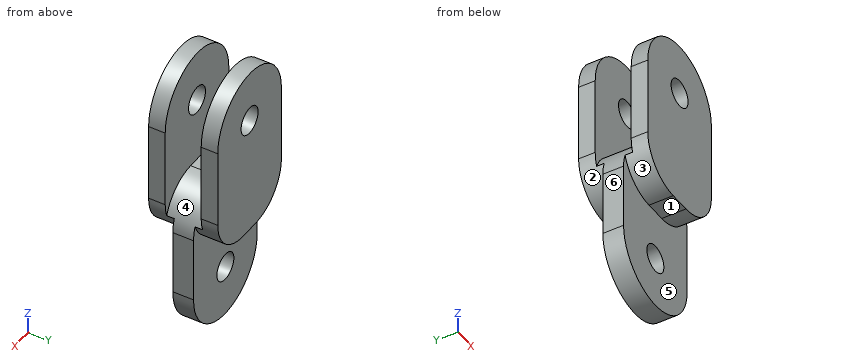
Autodesk Inventor part; units mm, degrees
ref_plane "YZ Plane" through (0, 0, 0) normal (1, 0, 0) x (0, 1, 0)
ref_plane "XZ Plane" through (0, 0, 0) normal (0, 1, 0) x (-1, 0, 0)
ref_plane "XY Plane" through (0, 0, 0) normal (0, 0, 1) x (1, 0, 0)
sketch "Sketch1" plane through (0, 0, 0) normal (0, 1, 0) x (-1, 0, 0)
  line L0 (7.5, 20) -> (-7.5, 20)
  line L1 (-7.5, 20) -> (-7.5, -20)
  line L2 (-7.5, -20) -> (7.5, -20)
  line L3 (7.5, -20) -> (7.5, 20)
  circle A0 centre (0, -12.5) radius 7.5
  circle A1 centre (0, 12.5) radius 7.5
  circle A2 centre (0, 12.5) radius 2
  circle A3 centre (0, -12.5) radius 2
  point P0 (0, 0)
  point P1 (7.5, 0)
  point P2 (0, -20)
  point P3 (7.5, 12.5)
  point P4 (-7.5, 12.5)
  point P5 (-7.5, -12.5)
  point P6 (7.5, -12.5)
  dimension "d0" = 15
  dimension "d2" = 25
  dimension "d3" = 4
  dimension "d4" = 4
extrude "Extrusion1" add sketch "Sketch1" along normal blind 10 contours A1 | L3 A0 L1 A1 | A0
sketch "Sketch2" plane through (7.5, 0, 12.5) normal (1, 0, 0) x (0, 0, -1)
  line L0 (-7.5, 0) -> (-7.5, 10)
  line L1 (-7.5, 7.6) -> (9.5, 7.6)
  line L2 (9.5, 7.6) -> (9.5, 2.4)
  line L3 (9.5, 2.4) -> (-7.5, 2.4)
  line L4 (-7.5, 2.4) -> (-7.5, 7.6)
  point P0 (12.5, 0)
  point P1 (-7.5, 5)
  point P2 (-7.5, 5)
  dimension "d7" = 17
  dimension "d8" = 5.2
extrude "Extrusion2" cut sketch "Sketch2" against normal through all
fillet "Fillet1" radius 6 2 edges at (7.5, 5, 3) (-7.5, 5, 3)
sketch "Sketch4" plane through (7.5, 0, 12.5) normal (1, 0, 0) x (0, 0, -1)
  line L0 (32.5, 0) -> (32.5, 10)
  line L1 (32.5, 6.5) -> (17.5, 6.5)
  line L2 (17.5, 6.5) -> (17.5, 3.5)
  line L3 (17.5, 3.5) -> (32.5, 3.5)
  line L4 (32.5, 3.5) -> (32.5, 6.5)
  line L5 (15.5, 2.4) -> (15.5, 7.6)
  line L6 (0, 0) -> (25, 0)
  line L7 (32.5, 3.5) -> (17.5, 3.5)
  line L8 (17.5, 3.5) -> (17.5, 0)
  line L9 (17.5, 0) -> (32.5, 0)
  line L10 (32.5, 0) -> (32.5, 3.5)
  line L11 (25, 10) -> (0, 10)
  line L12 (32.5, 6.5) -> (17.5, 6.5)
  line L13 (17.5, 6.5) -> (17.5, 10)
  line L14 (17.5, 10) -> (32.5, 10)
  line L15 (32.5, 10) -> (32.5, 6.5)
  point P0 (12.5, 0)
  point P1 (17.5, 5)
  point P2 (15.5, 5)
  point P3 (17.5, 1.75)
  dimension "d15" = 3
  dimension "d16" = 15
extrude "Extrusion4" cut sketch "Sketch4" against normal through all contours L9 L6 L8 L3 L0 | L1 L13 L11 L14 L0
fillet "Fillet2" radius 6 4 edges at (7.5, 1.75, -5) (7.5, 8.25, -5) (-7.5, 1.75, -5) (-7.5, 8.25, -5)
properties part number "coupler"
CAD build for the part. Positions are in the model's coordinates, mm. Face numbers are marked on the shaded views. A direction names the side the tool comes from. Round coordinates to 2 decimals unless told otherwise and drop trailing zeros. Loops run counter-clockwise (first coordinate to the right, second up) from the corner with the lowest first, then second, coordinate; pieces in that order, holes last.
(1) Wall check: line 1 along Z through (x, y) = (0, 0.9); line 2 along Y through (x, z) = (-3, 12.5); line 3 along X through (y, z) = (5.8, -12.5). Give the ranges that are in metal, low to high.
(2) Which spindle directions (+Z, -Z, +X, -X, +Y, -Y) get a long thin tool onto all of the face, cutting with end or side? Do the marked faces 1, 2 and 3. Say none if no direction does.
(3) Cut at A-A (x = 0). Give the cut face in (y, z).
(4) Two-plate mould, pull along Y, no slides. Class the marked faces 4, 5 and 6: +Y half, -Y half, draft (parallel to the pull), parting line (faces both ways), or undercut.
(5) Cut at D-D (x = -3.25). Give the cut face in (y, z), plus the area to 3 significant figures.
(6) Drop flat-ended pins along their axis: pin 1 (6 mm diameter, centred on x = 2.5, z = -13, fed in from -Y); pin 2 (1 mm diameter, centred on x = -5, z = -13, fed in from +Y); pin 3 (0.9 mm diameter, centred on x = 0.5, y = 2, fed in from -Z). Give the stop position or say it passes through.
(7) Cut at B-B (y = 8.75). Give the cut face in (x, z), plus the area to 3 significant figures.
(8) Cut at C-C (z = 4). Give the cut face in (x, y), plus the area to 3 significant figures.
Findings below:
1. line 1: z = -5 to 10.5, 14.5 to 20
1. line 2: y = 0 to 2.4, 7.6 to 10
1. line 3: x = -7.5 to -2, 2 to 7.5
2. face 1: -Z, +X, -X, -Y
2. face 2: -Z, -X, +Y
2. face 3: -Z, -X, -Y
3. outline: (0, -5) - (3.5, -5) - (3.5, -10.5) - (6.5, -10.5) - (6.5, -5) - (10, -5) - (10, 10.5) - (7.6, 10.5) - (7.6, 3) - (2.4, 3) - (2.4, 10.5) - (0, 10.5) - close; (0, 14.5) - (2.4, 14.5) - (2.4, 20) - (0, 20) - close; (3.5, -20) - (6.5, -20) - (6.5, -14.5) - (3.5, -14.5) - close; (7.6, 14.5) - (10, 14.5) - (10, 20) - (7.6, 20) - close
4. face 4: undercut
4. face 5: -Y half
4. face 6: draft
5. outline: (0, -4.74) - (3.5, -4.74) - (3.5, -19.26) - (6.5, -19.26) - (6.5, -4.74) - (10, -4.74) - (10, 19.26) - (7.6, 19.26) - (7.6, 2.74) - (2.4, 2.74) - (2.4, 19.26) - (0, 19.26) - close
5. area: 198 mm2
6. pin 1: stops at y = 3.5
6. pin 2: stops at y = 6.5
6. pin 3: stops at z = -5
7. outline: (-7.5, 1) arc R6 ccw to (-1.5, -5) - (1.5, -5) arc R6 ccw to (7.5, 1) - (7.5, 12.5) arc R7.5 ccw to (-7.5, 12.5) - close; hole circle Ø4 at (0, 12.5)
7. area: 323 mm2
8. outline: (-7.5, 0) - (7.5, 0) - (7.5, 2.4) - (-7.5, 2.4) - close; (-7.5, 7.6) - (7.5, 7.6) - (7.5, 10) - (-7.5, 10) - close
8. area: 72.0 mm2
